from build123d import *

# Parameters (mm, degrees)
BOSS_EXTRUDE1_DEPTH = 5
CUT_EXTRUDE1_REACH  = 7
SKETCH1_4_R         = 2
CUT_EXTRUDE2_DEPTH  = 5
BOSS_EXTRUDE2_DEPTH = 5
SKETCH6_R           = 2
CUT_EXTRUDE3_DEPTH  = 5


with BuildPart() as part:
    # Sketch1 → Boss-Extrude1 (new body)
    with BuildSketch(Plane.XY):
        with BuildLine():
            Line((-2.520114714, 12.269831909), (-0.124248164, 18.700029955))
            ThreePointArc((-0.124248164, 18.700029955), (0.116981353, 20.068110528), (-0.124248164, 21.436191102))
            Line((-0.124248164, 21.436191102), (-8.39066093, 29.702603869))
            Line((-8.39066093, 29.702603869), (2.215940787, 40.309205586))
            Line((2.215940787, 40.309205586), (2.215940787, 35.309205586))
            Line((2.215940787, 35.309205586), (5.841171936, 35.309205586))
            Line((5.841171936, 35.309205586), (5.841171936, 40.309205586))
            ThreePointArc((5.841171936, 40.309205586), (3.603256686, 43.658482445), (-0.347484741, 42.872631115))
            Line((-0.347484741, 42.872631115), (-10.954086459, 32.266029397))
            ThreePointArc((-10.954086459, 32.266029397), (-12.015892078, 29.702603869), (-10.954086459, 27.13917834))
            Line((-10.954086459, 27.13917834), (-3.883018647, 20.068110528))
            Line((-3.883018647, 20.068110528), (-8.158270438, 8.321952769))
            ThreePointArc((-8.158270438, 8.321952769), (0.921343905, 1.354919643), (-2.520114714, 12.269831909))
        make_face()
    extrude(amount=BOSS_EXTRUDE1_DEPTH)

    # Sketch1_4 → Cut-Extrude1 (cut, up to next)
    with BuildSketch(Plane.XY, mode=Mode.PRIVATE) as cut_extrude1_sk1:
        with Locations((-2.520114714, 6.269831909)):
            Circle(SKETCH1_4_R)
    cut_extrude1_tool1 = extrude(cut_extrude1_sk1.sketch, amount=CUT_EXTRUDE1_REACH, mode=Mode.PRIVATE) & part.part
    add(cut_extrude1_tool1.solids().sort_by_distance((-2.520115, 6.269832, 0))[0], mode=Mode.SUBTRACT)

    # Sketch5 → Cut-Extrude2 (cut)
    with BuildSketch(Plane(origin=(0, 0, 0), x_dir=(-1, 0, 0), z_dir=(0, 0, -1))):
        with BuildLine():
            Line((2.022476226, 12.24915929), (2.209173599, 10.005914968))
            ThreePointArc((2.209173599, 10.005914968), (-1.215968345, 5.958890794), (2.831055828, 2.53374885))
            Line((2.831055828, 2.53374885), (3.017753201, 0.290504527))
            ThreePointArc((3.017753201, 0.290504527), (-3.459212668, 5.772193421), (2.022476226, 12.24915929))
        make_face()
    extrude(amount=-CUT_EXTRUDE2_DEPTH, mode=Mode.SUBTRACT)

    # Sketch3 → Boss-Extrude2 (add)
    with BuildSketch(Plane.XY):
        with BuildLine():
            ThreePointArc((3.320342305, 7.644263358), (2.148599503, 7.913084677), (1.034423028, 7.461579551))
            ThreePointArc((1.034423028, 7.461579551), (0.758834569, 8.087383175), (0.37416263, 8.65272084))
            ThreePointArc((0.37416263, 8.65272084), (1.347484271, 9.358334814), (1.740439947, 10.494482662))
            ThreePointArc((1.740439947, 10.494482662), (1.571875447, 10.657954118), (1.397043733, 10.814704811))
            ThreePointArc((1.397043733, 10.814704811), (0.291074687, 10.343452688), (-0.344924962, 9.323280867))
            ThreePointArc((-0.344924962, 9.323280867), (-0.93571885, 9.667579802), (-1.579222127, 9.898843088))
            ThreePointArc((-1.579222127, 9.898843088), (-1.206537867, 11.041800891), (-1.556440997, 12.191937359))
            ThreePointArc((-1.556440997, 12.191937359), (-1.788898653, 12.225108819), (-2.022476226, 12.24915929))
            ThreePointArc((-2.022476226, 12.24915929), (-2.640228932, 11.217836019), (-2.555121505, 10.018668465))
            ThreePointArc((-2.555121505, 10.018668465), (-3.235457637, 9.949952219), (-3.891995873, 9.758806412))
            ThreePointArc((-3.891995873, 9.758806412), (-4.262301713, 10.90253701), (-5.221412546, 11.627349059))
            ThreePointArc((-5.221412546, 11.627349059), (-5.428972435, 11.517550152), (-5.632077174, 11.399713939))
            ThreePointArc((-5.632077174, 11.399713939), (-5.525653002, 10.202249956), (-4.751946644, 9.282127916))
            ThreePointArc((-4.751946644, 9.282127916), (-5.261959741, 8.826643761), (-5.680757645, 8.286100061))
            ThreePointArc((-5.680757645, 8.286100061), (-6.65260934, 8.99373724), (-7.854580137, 9.016371303))
            ThreePointArc((-7.854580137, 9.016371303), (-7.957961436, 8.805541479), (-8.053014233, 8.590828011))
            ThreePointArc((-8.053014233, 8.590828011), (-7.2630636, 7.684613857), (-6.096287842, 7.394992676))
            ThreePointArc((-6.096287842, 7.394992676), (-6.241170236, 6.726720077), (-6.262261243, 6.043247807))
            ThreePointArc((-6.262261243, 6.043247807), (-7.464444479, 6.044498216), (-8.450163248, 5.35630885))
            ThreePointArc((-8.450163248, 5.35630885), (-8.409877814, 5.124977936), (-8.360571733, 4.895400459))
            ThreePointArc((-8.360571733, 4.895400459), (-7.18882893, 4.62657914), (-6.074652455, 5.078084267))
            ThreePointArc((-6.074652455, 5.078084267), (-5.799063996, 4.452280642), (-5.414392057, 3.886942978))
            ThreePointArc((-5.414392057, 3.886942978), (-6.387713698, 3.181329004), (-6.780669374, 2.045181156))
            ThreePointArc((-6.780669374, 2.045181156), (-6.612104874, 1.881709699), (-6.43727316, 1.724959006))
            ThreePointArc((-6.43727316, 1.724959006), (-5.331304114, 2.196211129), (-4.695304465, 3.21638295))
            ThreePointArc((-4.695304465, 3.21638295), (-4.104510577, 2.872084015), (-3.4610073, 2.640820729))
            ThreePointArc((-3.4610073, 2.640820729), (-3.83369156, 1.497862927), (-3.48378843, 0.347726458))
            ThreePointArc((-3.48378843, 0.347726458), (-3.251330774, 0.314554999), (-3.017753201, 0.290504527))
            ThreePointArc((-3.017753201, 0.290504527), (-2.400000495, 1.321827799), (-2.485107922, 2.520995353))
            ThreePointArc((-2.485107922, 2.520995353), (-1.80477179, 2.589711598), (-1.148233554, 2.780857406))
            ThreePointArc((-1.148233554, 2.780857406), (-0.777927714, 1.637126807), (0.181183119, 0.912314758))
            ThreePointArc((0.181183119, 0.912314758), (0.388743008, 1.022113666), (0.591847747, 1.139949878))
            ThreePointArc((0.591847747, 1.139949878), (0.485423575, 2.337413862), (-0.288282783, 3.257535901))
            ThreePointArc((-0.288282783, 3.257535901), (0.221730314, 3.713020057), (0.640528217, 4.253563756))
            ThreePointArc((0.640528217, 4.253563756), (1.612379913, 3.545926577), (2.81435071, 3.523292514))
            ThreePointArc((2.81435071, 3.523292514), (2.917732009, 3.734122338), (3.012784806, 3.948835807))
            ThreePointArc((3.012784806, 3.948835807), (2.222834173, 4.855049961), (1.056058415, 5.144671141))
            ThreePointArc((1.056058415, 5.144671141), (1.200940809, 5.81294374), (1.222031815, 6.496416011))
            ThreePointArc((1.222031815, 6.496416011), (2.424215051, 6.495165601), (3.409933821, 7.183354967))
            ThreePointArc((3.409933821, 7.183354967), (3.369648387, 7.414685881), (3.320342305, 7.644263358))
        make_face()
    extrude(amount=BOSS_EXTRUDE2_DEPTH)

    # Sketch6 → Cut-Extrude3 (cut)
    with BuildSketch(Plane(origin=(0, 0, 0), x_dir=(-1, 0, 0), z_dir=(0, 0, -1))):
        with Locations((2.520114714, 6.269831909)):
            Circle(SKETCH6_R)
    extrude(amount=-CUT_EXTRUDE3_DEPTH, mode=Mode.SUBTRACT)


solid = part.part
Can you work these out from the model? Positions are in its coordinate system, mm. A direction names the side the tool comes from. Coordinates: 2 decimals unless noted, no trailing zeros. Write each loop counter-clockwise with the first axis right and the second up, starting at its lowest first coordinate (ties: lowest second). Pieces come first, ordered by that corner, then holes. Notation, with made-up numbers: M 55,18.5 L 65,18.5 A28 cw 65,36.5 Z; hole C 1,55.5 d2. An arc over 180 degrees is marked long. Use one line per item in the form item = value.
Q1. For P1, Ø1.5, axis at y = 38, z = 2, coming from the -X side; P2, Ø1.1, axis at x = 4.5, z = 3.5, coming from the -Y side, each with a flat end and sliding along its axis, tell me the tip position at first contact or that it passes through.
Model answer:
P1 = -5.97
P2 = 35.31
Q2. If we section it at B-B (y = 31): Write out the boundary of the cut face in (x, z), then the cut area to 3 significant figures.
Model answer:
outline = M -11.78,0 L -7.09,0 L -7.09,5 L -11.78,5 Z
area = 23.4 mm^2
Q3. We'd pull the mould along Y, two halves only. Please class faces 4 (the flat face through (-4, 24, 5)), 5 (the flat face through (-5.58, 37.64, 2.46)), 6 (the cylindrical face through (-1.207, 11.025, 2.465)): +Y half, -Y half, draft (parallel to the pull), parting line (faces both ways), or undercut.
Model answer:
face_4 = draft
face_5 = +Y half
face_6 = undercut
Q4. I need wall thicknesses on line 1 along Y through (x, z) = (-2.75, 3.5); line 2 along Y through (x, z) = (0.25, 1.6); line 3 along Y through (x, z) = (1.5, 4.85). Which ranges of each line are inside material? Lowest first, please. Write a range as from..to.
Model answer:
line_1 = 0.58..4.28, 8.26..24.06, 35.34..40.47
line_2 = 0.95..2.75, 3.74..10.31, 38.34..43.36
line_3 = 3.59..5.12, 6.43..7.75, 9.6..10.72, 39.59..43.86
Q5. For faces 1 (the flat face through (2.216, 38, 2)), 2 (the cylindrical face through (0.117, 20.049, 2.465)), 3 (the flat face through (-7.468, 23.653, 2.465)), which set-ups out of +Z, -Z, +X, -X, +Y, -Y let a thin tool reach every point of the face, with its end or its side?
Model answer:
face_1 = +Z, -Z
face_2 = +Z, -Z, +X
face_3 = +Z, -Z, -X
Q6. If we section it at C-C (x = 4.5): Write out the boundary of the cut face in (y, z), then the cut area to 3 significant figures.
Model answer:
outline = M 35.31,0 L 43.12,0 L 43.12,5 L 35.31,5 Z
area = 39.1 mm^2
Q7. If we section it at A-A (y = 36.5): Write out the boundary of the cut face in (x, z).
Model answer:
outline = M -6.72,0 L -1.59,0 L -1.59,5 L -6.72,5 Z; M 2.22,0 L 5.84,0 L 5.84,5 L 2.22,5 Z
